For this review, take the finished solid that the model builds, in its own axes (mm). Round coordinates to 2 decimals unless told otherwise and drop trailing zeros. Loops run counter-clockwise (first coordinate to the right, second up) from the corner with the lowest first, then second, coordinate; pieces in that order, holes last.
```python
from build123d import *

# Parameters (mm, degrees)
F1_DEPTH = 400


# Not quite as in the source:
# - a feature names something its author has since deleted; it is built from what else it names


with BuildPart() as f1:
    # F0 (on Front) → F1 (new body)
    with BuildSketch(Plane.XZ):
        Polygon((11.218088679, 20.9527928382), (11.218088679, 0), (28.4624192864, 0), (44.7796396911, 0), (28.4582051874, 20.9527928382), (28.2770004123, 28.9259795099), (-28.4582051874, 28.9259795099), (-28.4582051874, 20.9527928382), (-44.7796396911, 0), (-28.4624192864, 0), (-11.218088679, 0), (-11.218088679, 20.9527928382), align=None)
    extrude(amount=-F1_DEPTH)


solid = f1.part
```
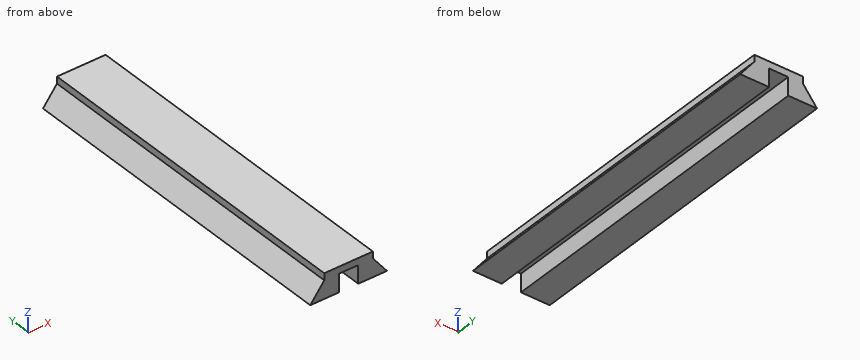
(1) Add section C-C (x = -37.5). Give the boundary of the cut face in (y, z), plus the area to 3 significant figures.
(2) For L1, parallel to X at y = 101.5, z = 9.5; L2, parallel to X at y = 256, z = 21; L3, parallel to Z at x = -36, y = 187, list the stretches that pass through material, from the lowest coordinate up.
(3) Add section B-B (y = 76). Give the boundary of the cut face in (x, z).
(4) Insertion check: pin 1 Ø2.5 at (y, z) = (224.5, 26) entering from -X; pin 2 Ø6.5 at (y, z) = (200.5, 13.5) entering from -X; pin 3 Ø1 at (y, z) = (212, 17.5) entering from -X; pin 4 Ø10 at (x, z) = (3, 15.5) entering from +Y. Each pin has a flat end and moves straight along its axis. Give the tip position at first contact, or say it passes through.
(5) Add section A-A (z = 13.75). Give the boundary of the cut face in (x, y).
Outcome:
1. outline: (0, 0) - (400, 0) - (400, 9.35) - (0, 9.35) - close
1. area: 3,740 mm2
2. L1: x = -37.38 to -11.22, 11.22 to 37.38
2. L2: x = -28.46 to 28.46
2. L3: z = 0 to 11.27
3. outline: (-44.78, 0) - (-11.22, 0) - (-11.22, 20.95) - (11.22, 20.95) - (11.22, 0) - (44.78, 0) - (28.46, 20.95) - (28.28, 28.93) - (-28.46, 28.93) - (-28.46, 20.95) - close
4. pin 1: stops at x = -28.46
4. pin 2: stops at x = -36.8
4. pin 3: stops at x = -31.54
4. pin 4: passes through
5. outline: (-34.07, 0) - (-11.22, 0) - (-11.22, 400) - (-34.07, 400) - close; (11.22, 0) - (34.07, 0) - (34.07, 400) - (11.22, 400) - close
